Autodesk Inventor part; units mm, degrees
ref_plane "YZ Plane" through (0, 0, 0) normal (1, 0, 0) x (0, 1, 0)
ref_plane "XZ Plane" through (0, 0, 0) normal (0, 1, 0) x (-1, 0, 0)
ref_plane "XY Plane" through (0, 0, 0) normal (0, 0, 1) x (1, 0, 0)
sketch "Эскиз1" plane through (0, 0, 0) normal (0, 0, 1) x (1, 0, 0)
  line L0 (0, 0) -> (0, 20)
  line L1 (0, 20) -> (2.8284, 22.8284)
  line L2 (0, 0) -> (15, 0)
  line L3 (15, 0) -> (15, 20)
  line L4 (15, 20) -> (12.1716, 22.8284)
  line L5 (12.1716, 22.8284) -> (2.8284, 22.8284)
  dimension "d0" = 20
  dimension "d1" = 4
  dimension "d2" = 135
  dimension "d3" = 15
  dimension "d4" = 4
  dimension "d5" = 135
revolve "Вращение1" add sketch "Эскиз1" angle 360 about axis through (0, 0, 0) along (1, 0, 0)
sketch "Эскиз2" plane through (0, 0, 0) normal (0, 0, 1) x (1, 0, 0)
  line L0 (15, -20) -> (15, 20)
  line L1 (15, 20) -> (10, 20)
  line L2 (10, 20) -> (10, 15)
  line L3 (10, 15) -> (15, 15)
  line L4 (15, 15) -> (15, 20)
  line L5 (15, 6) -> (10, 6)
  line L6 (10, 6) -> (10, 2)
  line L7 (10, 0) -> (15, 0)
  line L8 (15, 0) -> (15, 6)
  line L9 (10, 2) -> (6.8, 2)
  line L10 (6.8, 2) -> (6.8, 0)
  line L11 (6.8, 0) -> (10, 0)
  point P0 (0, 0)
  point P1 (15, 0)
  dimension "d7" = 5
  dimension "d8" = 5
  dimension "d9" = 6
  dimension "d10" = 2
  dimension "d11" = 5
  dimension "d12" = 3.2
revolve "Вращение2" cut sketch "Эскиз2" angle 360 about axis through (6.8, 0, 0) along (1, 0, 0)
sketch "Эскиз4" plane through (0, 0, 0) normal (1, 0, 0) x (0, 1, 0)
  point P0 (0, 0)
  point P1 (17, 0)
  dimension "d17" = 17
hole "Отверстие1" at (0, 17, 0) direction (1, 0, 0) diameter 3 depth 3 tip angle 90
sketch "Эскиз5" plane through (0, 0, 0) normal (0, 0, 1) x (1, 0, 0)
  line L0 (0, -20) -> (0, 20)
  line L1 (0, 2.5) -> (5.5, 2.5)
  line L2 (5.5, 2.5) -> (5.5, -2.5)
  line L3 (5.5, -2.5) -> (0, -2.5)
  line L4 (0, -2.5) -> (0, 2.5)
  point P0 (0, 0)
  point P1 (0, 0)
  point P2 (0, 0)
  dimension "d25" = 5
  dimension "d26" = 5.5
extrude "Выдавливание2" cut sketch "Эскиз5" along normal through all both and the other way through all
properties part number "711128"
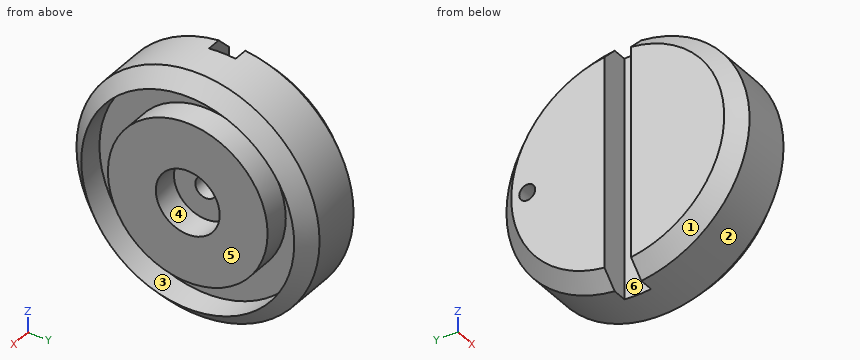
The listing builds one solid part. Answer for the finished solid, in the listing's coordinates (mm). Face numbers are marked on the shaded views. A direction names the side the tool comes from. Give positions to 0.01 mm unless a question says otherwise; leave off trailing zeros. Write each loop counter-clockwise with the first axis right and the second up, starting at its lowest first coordinate (ties: lowest second). Pieces come first, ordered by that corner, then holes. Notation, with made-up numbers: (76.5, 30.25) - (87.5, 30.25) arc R22 ccw to (87.5, 49.25) - close; hole circle Ø5 at (-29, -5.5). An arc over 180 degrees is marked (long way). One line per question, with ' | ' between items. Start each with the question number.
1. Straight lines are drawn through the part: line 1 (Z direction, x = 12.5, y = -13); line 2 (Z direction, x = 10.75, y = -2); line 3 (Z direction, x = 8.45, y = 0). For each, find the intervals that lie inside material, in ascending order.
2. Determine the mould class of the marked faces 1, 2 and 3 for opening direction Y: +Y half, -Y half, draft (parallel to the pull), parting line (faces both ways), or undercut.
3. Section B-B, the plane y = 0 is taken. Determine the outline of the cut face in (x, z).
4. Section C-C, the plane x = 2.25 is taken. Determine the outline of the cut face in (y, z).
5. Given P1, Ø14, axis at y = 0, z = 0, coming from the +X side; P2, Ø3, axis at y = 18, z = -12.5, coming from the -X side; P3, Ø2.5, axis at y = 17, z = 0, coming from the +X side; P4, Ø2, axis at x = 5.5, y = 6.5, coming from the -Z side, each flat-ended and moving along its own axis, determine where each tip first touches the part or whether it passes through.
6. For the marked faces 4, 5 and 6, determine the directions among +Z, -Z, +X, -X, +Y, -Y from which every point of the face is accessible in a straight line to the end or side of a thin tool.
7. Section A-A, the plane x = 10.75 is taken. Determine the outline of the cut face in (y, z).
Result:
1) line 1: z = -18.36 to -15.2, -7.48 to 7.48, 15.2 to 18.36 | line 2: z = -22.74 to -19.9, -14.87 to -5.66, 5.66 to 14.87, 19.9 to 22.74 | line 3: z = -22.83 to -2, 2 to 22.83
2) face 1: -Y half | face 2: parting line | face 3: undercut
3) outline: (5.5, -22.83) - (12.17, -22.83) - (15, -20) - (10, -20) - (10, -15) - (15, -15) - (15, -6) - (10, -6) - (10, -2) - (6.8, -2) - (6.8, 2) - (10, 2) - (10, 6) - (15, 6) - (15, 15) - (10, 15) - (10, 20) - (15, 20) - (12.17, 22.83) - (5.5, 22.83) - close
4) outline: (-2.5, -22.11) - (-2.5, 22.11) arc R22.25 ccw to start; (2.5, -22.11) arc R22.25 ccw to (2.5, 22.11) - close; hole circle Ø3 at (17, 0)
5) P1: stops at x = 15 | P2: stops at x = 0.41 | P3: stops at x = 10 | P4: stops at z = -22.16
6) face 4: +X | face 5: +Z, -Z, +X, +Y, -Y | face 6: +Z, -Z, -X
7) outline: circle Ø45.66 at (0, 0); circle Ø30 at (0, 0); hole circle Ø40 at (0, 0); hole circle Ø12 at (0, 0)
